Part model, mm, in its own coordinate system. A direction names the side the tool comes from. Give positions to 0.01 mm unless a question says otherwise; leave off trailing zeros. Order: outer loops, then holes, each group sorted by start corner. A loop starts at its lowest first (then second) coordinate and runs counter-clockwise, first axis right, second up. Notation, with made-up numbers: (3.5, -28.5) - (26.5, -28.5) arc R16 cw to (26.5, -4.5) - close; hole circle Ø3 at (73, 84.25). An arc over 180 degrees is marked (long way). Use one line per item in the form item = value. Start each with the question number.
1. Pin check, flat tips, straight feed: P1, Ø4, axis at x = 145.5, z = 1.5, coming from the +Y side; P2, Ø0.5, axis at x = 189.5, y = -0.5, coming from the -Z side; P3, Ø1.6, axis at y = 10, z = -40, coming from the +X side; P4, Ø3, axis at x = 2.32, y = 13, coming from the -Z side. Stop position of each tip, or through.
2. Band-saw the part on A-A, the plane y = 7.25. List the corners of the cut face in (x, z).
3. Band-saw the part on B-B, the plane x = 117. List the corners of the cut face in (y, z).
4. Drill centre lines: line 1 (X direction, y = 13, z = 44.1); line 2 (Z direction, x = 167, y = 4); line 3 (Y direction, x = 165, z = 22). Where is each one in solid material? Low to high.
5. Tool access for faces 5 (the face through (56, 0, 1)), 6 (the face through (56, 12, 44.801)): list every direction of +Z, -Z, +X, -X, +Y, -Y with a clear straight run to the whole face (end or side of a thin tool).
6. Pull direction Z, two halves, no side cores. Call faces 1 (the face through (59.4, 11.6, -41.199)), 2 (the face through (56, -1, 1)), 3 (the face through (59.4, 11.9, -40.199)), 4 (the face through (56, 12, 43.801)): +Z half, -Z half, draft (parallel to the pull), parting line (faces both ways), or undercut.
7. Band-saw the part on C-C, the plane z = 28. List the corners of the cut face in (x, y), plus the area to 3 significant figures.
from build123d import *

# Parameters (mm, degrees)
SKETCH1_W                      = 272
SKETCH1_H                      = 84
BASE_FLANGE1_DEPTH             = 1
EDGE_FLANGE1_STRIP_W           = 5
EDGE_FLANGE1_STRIP_H           = 1
EDGE_FLANGE1_STRIP_CUT_DEPTH   = 272
EDGE_FLANGE1_STRIP_2_W         = 5
EDGE_FLANGE1_STRIP_2_H         = 1
EDGE_FLANGE1_STRIP_CUT_2_DEPTH = 272
EDGE_FLANGE1_DEPTH             = 272
EDGE_FLANGE1_BEND_DEPTH        = 272
CUT_EXTRUDE1_START             = -78.427547771
CUT_EXTRUDE1_DEPTH             = 8.5
CUT_EXTRUDE1_START_2           = 185.072452229
CUT_EXTRUDE1_2_DEPTH           = 8.5
SKETCH13_R                     = 1.6
CUT_EXTRUDE2_DEPTH             = 100
SKETCH14_R                     = 1.5
CUT_EXTRUDE3_DEPTH             = 100
FILLET1_R                      = 2
FILLET2_R                      = 2
FILLET3_R                      = 2
FILLET4_R                      = 2
FILLET5_R                      = 2
FILLET6_R                      = 2
FILLET7_R                      = 2
FILLET8_R                      = 2


# Read off the part's stored shape, not the designer's step: Cut-Extrude1
# Sheet-metal steps are written as plain solids
with BuildPart() as part:
    # Sketch1 → Base-Flange1 (new body)
    with BuildSketch(Plane(origin=(0, 0, 0), x_dir=(1, 0, 0), z_dir=(0, 1, 0))):
        with Locations((57.572452229, -1.800955414)):
            Rectangle(SKETCH1_W, SKETCH1_H)
    extrude(amount=-BASE_FLANGE1_DEPTH)

    # Edge-Flange1 strip (across the edge) → Edge-Flange1 strip cut (cut)
    with BuildSketch(Plane(origin=(-78.427547771, 0, 43.800955414), x_dir=(0, 0, -1), z_dir=(1, 0, 0))):
        with Locations((-2, -0.5)):
            Rectangle(EDGE_FLANGE1_STRIP_W, EDGE_FLANGE1_STRIP_H)
    extrude(amount=EDGE_FLANGE1_STRIP_CUT_DEPTH, mode=Mode.SUBTRACT)

    # Edge-Flange1 strip 2 (across the edge) → Edge-Flange1 strip cut 2 (cut)
    with BuildSketch(Plane(origin=(193.572452229, 0, -40.199044586), x_dir=(0, 0, 1), z_dir=(-1, 0, 0))):
        with Locations((-2, -0.5)):
            Rectangle(EDGE_FLANGE1_STRIP_2_W, EDGE_FLANGE1_STRIP_2_H)
    extrude(amount=EDGE_FLANGE1_STRIP_CUT_2_DEPTH, mode=Mode.SUBTRACT)

    # Edge-Flange1 section (across the edge) → Edge-Flange1 (add)
    with BuildSketch(Plane(origin=(-78.427547771, 0, 43.800955414), x_dir=(0, 0, -1), z_dir=(1, 0, 0))):
        with BuildLine():
            Line((-1, 0.5), (-1, 23))
            Line((-1, 23), (0, 23))
            Line((0, 23), (0, 0.5))
            ThreePointArc((0, 0.5), (0.146446609, 0.146446609), (0.5, 0))
            Line((0.5, 0), (0.5, -1))
            ThreePointArc((0.5, -1), (-0.560660172, -0.560660172), (-1, 0.5))
        make_face()
    extrude(amount=EDGE_FLANGE1_DEPTH)

    # Edge-Flange1 section 2 (across the edge) → Edge-Flange1 bend (add)
    with BuildSketch(Plane(origin=(193.572452229, 0, -40.199044586), x_dir=(0, 0, 1), z_dir=(-1, 0, 0))):
        with BuildLine():
            Line((-1, 0.5), (-1, 23))
            Line((-1, 23), (0, 23))
            Line((0, 23), (0, 0.5))
            ThreePointArc((0, 0.5), (0.146446609, 0.146446609), (0.5, 0))
            Line((0.5, 0), (0.5, -1))
            ThreePointArc((0.5, -1), (-0.560660172, -0.560660172), (-1, 0.5))
        make_face()
    extrude(amount=EDGE_FLANGE1_BEND_DEPTH)

    # Cut-Extrude1 outline → Cut-Extrude1 (cut)
    with BuildSketch(Plane.YZ.offset(CUT_EXTRUDE1_START)):
        with BuildLine():
            ThreePointArc((0.5, -40.199044586), (0.146446609, -40.052597977), (0, -39.699044586))
            Line((0, -39.699044586), (-1, -39.699044586))
            ThreePointArc((-1, -39.699044586), (-0.560660172, -40.759704758), (0.5, -41.199044586))
            Line((0.5, -41.199044586), (23, -41.199044586))
            Line((23, -41.199044586), (23, -40.199044586))
            Line((23, -40.199044586), (0.5, -40.199044586))
        make_face()
        with BuildLine():
            ThreePointArc((0.5, 44.800955414), (-0.560660172, 44.361615586), (-1, 43.300955414))
            Line((-1, 43.300955414), (0, 43.300955414))
            ThreePointArc((0, 43.300955414), (0.146446609, 43.654508805), (0.5, 43.800955414))
            Line((0.5, 43.800955414), (23, 43.800955414))
            Line((23, 43.800955414), (23, 44.800955414))
            Line((23, 44.800955414), (0.5, 44.800955414))
        make_face()
    extrude(amount=CUT_EXTRUDE1_DEPTH, mode=Mode.SUBTRACT)

    # Cut-Extrude1 2 outline → Cut-Extrude1 2 (cut)
    with BuildSketch(Plane.YZ.offset(CUT_EXTRUDE1_START_2)):
        with BuildLine():
            ThreePointArc((0.5, -40.199044586), (0.146446609, -40.052597977), (0, -39.699044586))
            Line((0, -39.699044586), (-1, -39.699044586))
            ThreePointArc((-1, -39.699044586), (-0.560660172, -40.759704758), (0.5, -41.199044586))
            Line((0.5, -41.199044586), (23, -41.199044586))
            Line((23, -41.199044586), (23, -40.199044586))
            Line((23, -40.199044586), (0.5, -40.199044586))
        make_face()
        with BuildLine():
            ThreePointArc((0.5, 44.800955414), (-0.560660172, 44.361615586), (-1, 43.300955414))
            Line((-1, 43.300955414), (0, 43.300955414))
            ThreePointArc((0, 43.300955414), (0.146446609, 43.654508805), (0.5, 43.800955414))
            Line((0.5, 43.800955414), (23, 43.800955414))
            Line((23, 43.800955414), (23, 44.800955414))
            Line((23, 44.800955414), (0.5, 44.800955414))
        make_face()
    extrude(amount=CUT_EXTRUDE1_2_DEPTH, mode=Mode.SUBTRACT)

    # Sketch13 → Cut-Extrude2 (cut)
    with BuildSketch(Plane(origin=(0, 0, -41.199044586), x_dir=(-1, 0, 0), z_dir=(0, 0, -1))):
        with Locations(Location((-168.072452229, 13, 0), (0, 0, 90))):
            Circle(SKETCH13_R)
        with Locations(Location((-112.822452229, 13, 0), (0, 0, 90))):
            Circle(SKETCH13_R)
        with Locations(Location((-57.572452229, 13, 0), (0, 0, 90))):
            Circle(SKETCH13_R)
        with Locations(Location((-2.322452229, 13, 0), (0, 0, 90))):
            Circle(SKETCH13_R)
        with Locations(Location((52.927547771, 13, 0), (0, 0, 90))):
            Circle(SKETCH13_R)
    extrude(amount=-CUT_EXTRUDE2_DEPTH, mode=Mode.SUBTRACT)

    # Sketch14 → Cut-Extrude3 (cut)
    with BuildSketch(Plane(origin=(0, 0, 0), x_dir=(1, 0, 0), z_dir=(0, 1, 0))):
        with Locations(Location((-74.427547771, -1.800955414, 0), (0, 0, 270))):
            Circle(SKETCH14_R)
        with Locations(Location((-74.427547771, 32.199044586, 0), (0, 0, 270))):
            Circle(SKETCH14_R)
        with Locations(Location((-74.427547771, -35.800955414, 0), (0, 0, 270))):
            Circle(SKETCH14_R)
        with Locations(Location((189.572452229, -35.800955414, 0), (0, 0, 270))):
            Circle(SKETCH14_R)
        with Locations(Location((189.572452229, -1.800955414, 0), (0, 0, 270))):
            Circle(SKETCH14_R)
        with Locations(Location((189.572452229, 32.199044586, 0), (0, 0, 270))):
            Circle(SKETCH14_R)
    extrude(amount=-CUT_EXTRUDE3_DEPTH, mode=Mode.SUBTRACT)

    # Fillet1
    fillet1_edges = [part.edges().sort_by_distance(p)[0] for p in [
        (193.572452229, -0.5, -39.699044586),
    ]]
    fillet(fillet1_edges, radius=FILLET1_R)

    # Fillet2
    fillet2_edges = [part.edges().sort_by_distance(p)[0] for p in [
        (193.572452229, -0.5, 43.300955414),
    ]]
    fillet(fillet2_edges, radius=FILLET2_R)

    # Fillet3
    fillet3_edges = [part.edges().sort_by_distance(p)[0] for p in [
        (-78.427547771, -0.5, -39.699044586),
    ]]
    fillet(fillet3_edges, radius=FILLET3_R)

    # Fillet4
    fillet4_edges = [part.edges().sort_by_distance(p)[0] for p in [
        (-78.427547771, -0.5, 43.300955414),
    ]]
    fillet(fillet4_edges, radius=FILLET4_R)

    # Fillet5
    fillet5_edges = [part.edges().sort_by_distance(p)[0] for p in [
        (185.072452229, 23, -40.699044586),
    ]]
    fillet(fillet5_edges, radius=FILLET5_R)

    # Fillet6
    fillet6_edges = [part.edges().sort_by_distance(p)[0] for p in [
        (-69.927547771, 23, -40.699044586),
    ]]
    fillet(fillet6_edges, radius=FILLET6_R)

    # Fillet7
    fillet7_edges = [part.edges().sort_by_distance(p)[0] for p in [
        (185.072452229, 23, 44.300955414),
    ]]
    fillet(fillet7_edges, radius=FILLET7_R)

    # Fillet8
    fillet8_edges = [part.edges().sort_by_distance(p)[0] for p in [
        (-69.927547771, 23, 44.300955414),
    ]]
    fillet(fillet8_edges, radius=FILLET8_R)


solid = part.part
From the geometry:
q1.P1 = 0
q1.P2 = -39.7
q1.P3 = 185.07
q1.P4 = through
q2.outline = (-69.93, -41.2) - (185.07, -41.2) - (185.07, -40.2) - (-69.93, -40.2) - close; (-69.93, 43.8) - (185.07, 43.8) - (185.07, 44.8) - (-69.93, 44.8) - close
q3.outline = (-1, -39.7) arc R1.5 ccw to (0.5, -41.2) - (23, -41.2) - (23, -40.2) - (0.5, -40.2) arc R0.5 cw to (0, -39.7) - (0, 43.3) arc R0.5 cw to (0.5, 43.8) - (23, 43.8) - (23, 44.8) - (0.5, 44.8) arc R1.5 ccw to (-1, 43.3) - close
q4.line_1 = -69.93 to -54.53, -51.33 to 0.72, 3.92 to 55.97, 59.17 to 111.22, 114.42 to 166.47, 169.67 to 185.07
q4.line_2 = -41.2 to -40.2, 43.8 to 44.8
q4.line_3 = -1 to 0
q5.face_5 = +X, -X, +Y
q5.face_6 = +Z, +X, -X, +Y, -Y
q6.face_1 = -Z half
q6.face_2 = draft
q6.face_3 = undercut
q6.face_4 = undercut
q7.outline = (-78.43, -1) - (193.57, -1) - (193.57, 0) - (-78.43, 0) - close
q7.area = 272 mm²
